Answer from the drawing. Dimensions are ordinates in mm from the lowest x, y and z of the part. A direction names the side the tool comes from. Coordinates: 2 decimals unless noted, no trailing zeros. Order: outer loops, then holes, each group sorted by start corner. A loop starts at its lowest first (then second) coordinate and runs counter-clockwise, first axis right, second up.
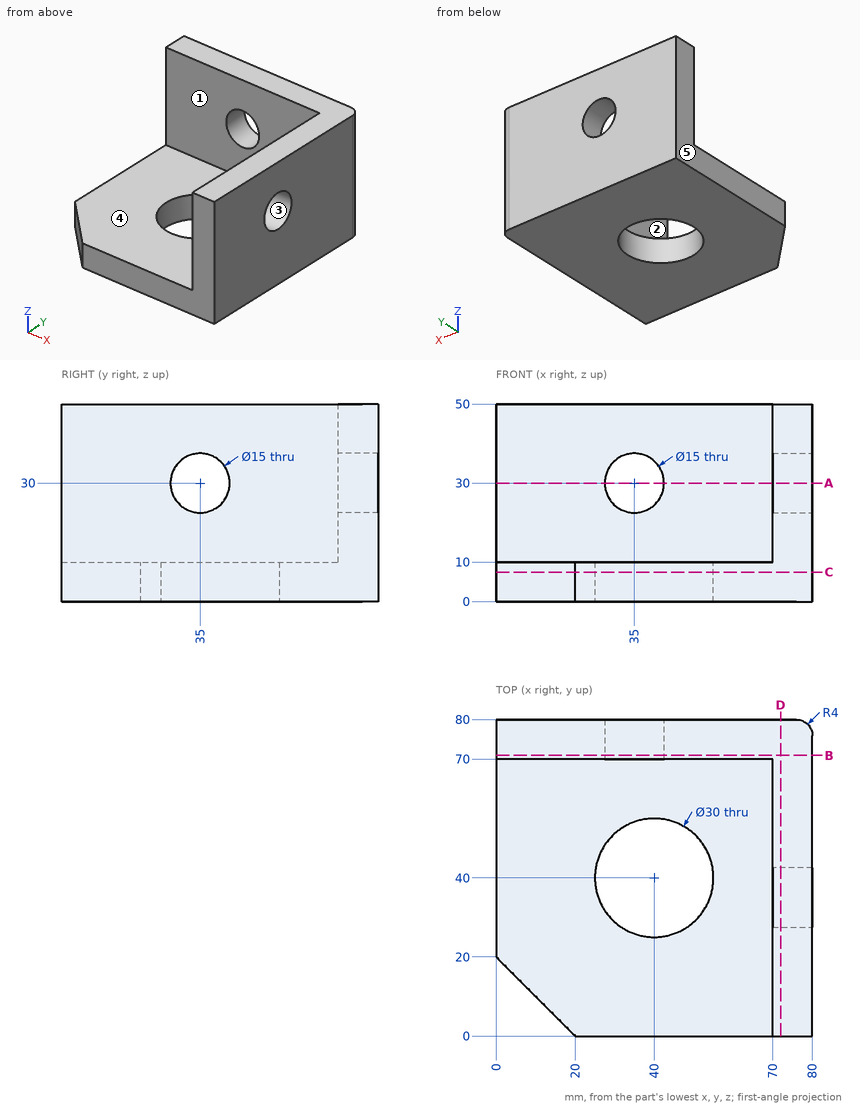
1) Each of these flat-tipped pins is pushed along its axis until it touches: P1, Ø2, axis at x = 44.5, z = 30.5, coming from the -Y side; P2, Ø12, axis at y = 46, z = 33.5, coming from the -X side; P3, Ø2, axis at x = 64, y = 37.5, coming from the +Z side. Where does it stop, or does it pass through?
2) Consider L1, parallel to Z at x = 74.5, y = 35; L2, parallel to Y at x = 40, z = 5.75; L3, parallel to Z at x = 14.5, y = 31. Determine where each line is inside the solid, lowest interval first.
3) Determine the mould class of the marked faces 1, 2 and 3 for opening direction Y: released by +Y, released by -Y, zero draft, split by the parting line, or undercut.
4) Section C-C (z = 7.5) is taken. Give the vertices of the cut face in (x, y), then the cut area to 3 significant figures.
5) Section A-A (z = 30) is taken. Give the vertices of the cut face in (x, y).
6) Section B-B (y = 71) is taken. Give the vertices of the cut face in (x, z), then the cut area to 3 significant figures.
7) A tool of negligible diameter and unlimited length cuts with its end or side. For the marked faces 4 and 5, from which of +Z, -Z, +X, -X, +Y, -Y can it reach the whole face along a straight path? Write none if from no direction.
Filled sheet:
1. P1: stops at y = 70
1. P2: stops at x = 70
1. P3: stops at z = 10
2. L1: z = 0 to 22.5, 37.5 to 50
2. L2: y = 0 to 25, 55 to 80
2. L3: z = 0 to 10
3. face 1: released by -Y
3. face 2: zero draft
3. face 3: undercut
4. outline: (0, 20) - (20, 0) - (80, 0) - (80, 76) arc R4 ccw to (76, 80) - (0, 80) - close; hole circle Ø30 at (40, 40)
4. area: 5,490 mm2
5. outline: (0, 70) - (27.5, 70) - (27.5, 80) - (0, 80) - close; (42.5, 70) - (70, 70) - (70, 42.5) - (80, 42.5) - (80, 76) arc R4 ccw to (76, 80) - (42.5, 80) - close; (70, 0) - (80, 0) - (80, 27.5) - (70, 27.5) - close
6. outline: (0, 0) - (80, 0) - (80, 50) - (0, 50) - close; hole circle Ø15 at (35, 30)
6. area: 3,820 mm2
7. face 4: +Z, -X, -Y
7. face 5: +Z, -Z, -X, +Y, -Y
